from build123d import *

# Parameters (mm, degrees)
SALIENTE_EXTRUIR1_DEPTH = 20
SALIENTE_EXTRUIR2_DEPTH = 4
REDONDEO1_R             = 1
REDONDEO2_R             = 10
CROQUIS3_R              = 1.8
CORTAR_EXTRUIR1_DEPTH   = 6
CROQUIS4_R              = 1.8
CORTAR_EXTRUIR2_DEPTH   = 6
CROQUIS5_R              = 3.2
CORTAR_EXTRUIR3_DEPTH   = 4
CROQUIS6_R              = 3.2
CORTAR_EXTRUIR4_DEPTH   = 4


with BuildPart() as part:
    # Croquis2 → Saliente-Extruir1 (new body)
    with BuildSketch(Plane.XY):
        Polygon((0, 0), (-17.960512242, 17.960512242), (-17.960512242, 9.475230868), (0, -8.485281374), align=None)
        Polygon((0, -8.485281374), (0, 0), (17.960512242, 17.960512242), (17.960512242, 9.475230868), align=None)
    extrude(amount=-SALIENTE_EXTRUIR1_DEPTH)

    # Croquis2<3> → Saliente-Extruir2 (add)
    with BuildSketch(Plane.XY):
        Polygon((0, 0), (-17.960512242, 17.960512242), (-17.960512242, 9.475230868), (0, -8.485281374), align=None)
        with BuildLine():
            Line((-17.960512242, 17.960512242), (0, 0))
            Line((0, 0), (0, 10.760512242))
            ThreePointArc((0, 10.760512242), (-5.091168825, 12.869343418), (-7.2, 17.960512242))
            ThreePointArc((-7.2, 17.960512242), (-10, 15.160512242), (-12.8, 17.960512242))
            Line((-12.8, 17.960512242), (-12.8, 67.960512242))
            ThreePointArc((-12.8, 67.960512242), (-12.796319785, 68.104024126), (-12.785288814, 68.247158756))
            Line((-12.785288814, 68.247158756), (-17.960512242, 17.960512242))
        make_face()
        with BuildLine():
            Line((0, 10.760512242), (0, 0))
            Line((0, 0), (17.960512242, 17.960512242))
            Line((17.960512242, 17.960512242), (12.785288814, 68.247158756))
            ThreePointArc((12.785288814, 68.247158756), (12.796319785, 68.104024126), (12.8, 67.960512242))
            Line((12.8, 67.960512242), (12.8, 17.960512242))
            ThreePointArc((12.8, 17.960512242), (10, 15.160512242), (7.2, 17.960512242))
            ThreePointArc((7.2, 17.960512242), (5.091168825, 12.869343418), (0, 10.760512242))
        make_face()
        Polygon((0, -8.485281374), (0, 0), (17.960512242, 17.960512242), (17.960512242, 9.475230868), align=None)
        with BuildLine():
            Line((12.8, 67.960512242), (12.8, 17.960512242))
            ThreePointArc((12.8, 17.960512242), (10, 15.160512242), (7.2, 17.960512242))
            Line((7.2, 17.960512242), (7.2, 67.960512242))
            ThreePointArc((7.2, 67.960512242), (10, 70.760512242), (12.8, 67.960512242))
        make_face()
        with BuildLine():
            ThreePointArc((11.5, 67.960512242), (10, 69.460512242), (8.5, 67.960512242))
            Line((8.5, 67.960512242), (8.5, 17.960512242))
            ThreePointArc((8.5, 17.960512242), (10, 16.460512242), (11.5, 17.960512242))
            Line((11.5, 17.960512242), (11.5, 67.960512242))
        make_face(mode=Mode.SUBTRACT)
        with BuildLine():
            ThreePointArc((-12.8, 67.960512242), (-10, 70.760512242), (-7.2, 67.960512242))
            Line((-7.2, 67.960512242), (-7.2, 17.960512242))
            ThreePointArc((-7.2, 17.960512242), (-10, 15.160512242), (-12.8, 17.960512242))
            Line((-12.8, 17.960512242), (-12.8, 67.960512242))
        make_face()
        with BuildLine():
            Line((-11.5, 67.960512242), (-11.5, 17.960512242))
            ThreePointArc((-11.5, 17.960512242), (-10, 16.460512242), (-8.5, 17.960512242))
            Line((-8.5, 17.960512242), (-8.5, 67.960512242))
            ThreePointArc((-8.5, 67.960512242), (-10, 69.460512242), (-11.5, 67.960512242))
        make_face(mode=Mode.SUBTRACT)
        with BuildLine():
            ThreePointArc((-10, 70.760512242), (-8.020101013, 69.940411229), (-7.2, 67.960512242))
            Line((-7.2, 67.960512242), (0, 67.960512242))
            Line((0, 67.960512242), (0, 70.760512242))
            Line((0, 70.760512242), (-10, 70.760512242))
        make_face()
        with BuildLine():
            ThreePointArc((7.2, 67.960512242), (8.020101013, 69.940411229), (10, 70.760512242))
            Line((10, 70.760512242), (0, 70.760512242))
            Line((0, 70.760512242), (0, 67.960512242))
            Line((0, 67.960512242), (7.2, 67.960512242))
        make_face()
    extrude(amount=SALIENTE_EXTRUIR2_DEPTH)

    # Redondeo1
    redondeo1_edges = [part.edges().sort_by_distance(p)[0] for p in [
        (-8.980256121, 8.980256121, 0),
        (8.980256121, 8.980256121, 0),
    ]]
    fillet(redondeo1_edges, radius=REDONDEO1_R)

    # Redondeo2
    redondeo2_edges = [part.edges().sort_by_distance(p)[0] for p in [
        (0, -8.485281374, -8),
    ]]
    fillet(redondeo2_edges, radius=REDONDEO2_R)

    # Croquis3 → Cortar-Extruir1 (cut)
    with BuildSketch(Plane(origin=(0, 0, 0), x_dir=(0, 0, -1), z_dir=(0.707106781, 0.707106781, 0))):
        with Locations((14, 12.7)):
            Circle(CROQUIS3_R)
    extrude(amount=-CORTAR_EXTRUIR1_DEPTH, mode=Mode.SUBTRACT)

    # Croquis4 → Cortar-Extruir2 (cut)
    with BuildSketch(Plane(origin=(0, 0, 0), x_dir=(0, 0, 1), z_dir=(-0.707106781, 0.707106781, 0))):
        with Locations((-14, 12.7)):
            Circle(CROQUIS4_R)
    extrude(amount=-CORTAR_EXTRUIR2_DEPTH, mode=Mode.SUBTRACT)

    # Croquis5 → Cortar-Extruir3 (cut)
    with BuildSketch(Plane(origin=(4.242640687, -4.242640687, 0), x_dir=(0, 0, -1), z_dir=(0.707106781, -0.707106781, 0))):
        with Locations((14, 12.7)):
            Circle(CROQUIS5_R)
    extrude(amount=-CORTAR_EXTRUIR3_DEPTH, mode=Mode.SUBTRACT)

    # Croquis6 → Cortar-Extruir4 (cut)
    with BuildSketch(Plane(origin=(-4.242640687, -4.242640687, 0), x_dir=(0, 0, 1), z_dir=(-0.707106781, -0.707106781, 0))):
        with Locations((-14, 12.7)):
            Circle(CROQUIS6_R)
    extrude(amount=-CORTAR_EXTRUIR4_DEPTH, mode=Mode.SUBTRACT)


solid = part.part
Check sheet for the modelled part. Datum: model origin and axes. Units: mm. A direction names the side the tool comes from. Give positions to 0.01 mm unless a question says otherwise; leave off trailing zeros. Write each loop counter-clockwise with the first axis right and the second up, starting at its lowest first coordinate (ties: lowest second). Pieces come first, ordered by that corner, then holes. Notation, with made-up numbers: (66.25, 10) -> (71.25, 10) arc R12 cw to (71.25, 16) -> close; hole circle Ø9 at (-25, 47). An arc over 180 degrees is marked (long way). Use one line per item in the form item = value. Start each with the question number.
1. Section check B-B (y = 57). Record the cut outline in (x, z), and give its area (3 significant figures).
2. Mould release check, pull along Y, two halves, no side actions. Record for faces 1 (the cylindrical face through (-9.196, 9.599, -0.301)), 2 (the cylindrical face through (10.03, 69.46, 1.97)), 3 (the flat face through (8, 25, 4)): pulls with the +Y half, pulls with the -Y half, needs draft (parallel to the pull), parting line crosses it, or undercut.
3. Access from +Z, -Z, +X, -X, +Y, -Y to the whole of each face (thin tool, end or side, straight path). Record for faces 4 (the cylindrical face through (9.185, 9.61, -0.285)), 5 (the cylindrical face through (-11.9, 6.2, -17.2)), 6 (the flat face through (11.5, 43, 2)).
4. Thickness scan on line 1 along X through (y, z) = (38, 2.5); line 2 along Z through (x, y) = (8, 47); line 3 along X through (y, z) = (13.5, -4.75). Record the ranges inside material, lowest first. Write a range as from..to.
5. Go/stop test with flat-tipped pins: P1, Ø18, axis at x = -2.5, y = 42, coming from the -Z side; P2, Ø3, axis at y = 40, z = 2, coming from the +X side; P3, Ø10, axis at y = 3.5, z = -4, coming from the +X side. Record where each tip stops, or that it passes through.
6. Section check A-A (z = -15). Record the cut outline in (x, y).
Conclusion:
q1.outline = (-13.94, 0) -> (-11.5, 0) -> (-11.5, 4) -> (-13.94, 4) -> close; (-8.5, 0) -> (-7.2, 0) -> (-7.2, 4) -> (-8.5, 4) -> close; (7.2, 0) -> (8.5, 0) -> (8.5, 4) -> (7.2, 4) -> close; (11.5, 0) -> (13.94, 0) -> (13.94, 4) -> (11.5, 4) -> close
q1.area = 29.9 mm²
q2.face_1 = pulls with the +Y half
q2.face_2 = undercut
q2.face_3 = needs draft
q3.face_4 = -Z, +Y
q3.face_5 = none
q3.face_6 = +Z, -Z
q4.line_1 = -15.9..-11.5, -8.5..-7.2, 7.2..8.5, 11.5..15.9
q4.line_2 = 0..4
q4.line_3 = -17.96..-13.5, 13.5..17.96
q5.P1 = 0
q5.P2 = 15.85
q5.P3 = 16.99
q6.outline = (-17.96, 9.48) -> (-15.37, 6.89) -> (-12.54, 9.72) -> (-11.45, 8.62) -> (-10.04, 10.04) -> (-17.96, 17.96) -> close; (-11.07, 2.59) -> (-7.07, -1.41) arc R10 ccw to (7.07, -1.41) -> (11.07, 2.59) -> (8.25, 5.42) -> (9.34, 6.51) -> (7.92, 7.92) -> (0, 0) -> (-7.92, 7.92) -> (-9.34, 6.51) -> (-8.25, 5.42) -> close; (10.04, 10.04) -> (11.45, 8.62) -> (12.54, 9.72) -> (15.37, 6.89) -> (17.96, 9.48) -> (17.96, 17.96) -> close
